Read the model definition and answer for the solid it produces. Units are mm, in the model's axes. Round coordinates to 2 decimals unless told otherwise and drop trailing zeros. Order: outer loops, then holes, each group sorted by start corner. A loop starts at its lowest first (then second) coordinate and runs counter-clockwise, first axis right, second up. Notation, with made-up numbers: (-12.75, 53.5) -> (45.25, 53.5) arc R12 cw to (45.25, 58.5) -> close; hole circle Ø9 at (36, -36.75). An arc over 180 degrees is marked (long way). Answer as a JSON object with one key per item and string values. Group by question number.
Item 1: Given P1, Ø2, axis at x = 2, z = 17.5, coming from the +Y side, flat-ended and moving along its own axis, determine where the tip first touches the part or whether it passes through.
Item 2: Section C-C, the plane z = 13.25 is taken. Write down the section's boundary in (x, y).
Item 3: Consider probe 1 along Z at (x, y) = (9, 52.5); probe 2 along Y at (x, z) = (9.25, 19.75); probe 3 along Z at (x, y) = (2.75, 44.25). Determine where each line is inside the solid, lowest interval first. Write a range as from..to.
Item 4: Section A-A, the plane y = 46 is taken. Write down the section's boundary in (x, z).
Item 5: Section B-B, the plane x = 2.5 is taken. Write down the section's boundary in (y, z), plus the area to 3 significant figures.
from build123d import *

# Parameters (mm, degrees)
F0_R     = 10.177589
F1_DEPTH = 11.176
F2_R     = 10.040254
F3_DEPTH = 11.176


with BuildPart() as f1:
    # F0 (on Right) → F1 (new body)
    with BuildSketch(Plane.YZ):
        with Locations((47.875904, 10.407805)):
            Circle(F0_R)
    extrude(amount=F1_DEPTH)


with BuildPart() as f3:
    # F2 (on Right) → F3 (new body)
    with BuildSketch(Plane.YZ):
        with Locations((-41.587934, 10.073202)):
            Circle(F2_R)
    extrude(amount=F3_DEPTH)


solid = f1.part
Values found:
{
 "1": {"P1": "y = 56.03"},
 "2": {"outline": "(0, 38.1) -> (11.18, 38.1) -> (11.18, 57.65) -> (0, 57.65) -> close"},
 "3": {"probe 1": "1.34..19.47", "probe 2": "43.84..51.91", "probe 3": "0.9..19.92"},
 "4": {"outline": "(0, 0.4) -> (11.18, 0.4) -> (11.18, 20.41) -> (0, 20.41) -> close"},
 "5": {"outline": "circle Ø20.36 at (47.88, 10.41)", "area": "325 mm2"}
}
